Build history of the part. All positions in model axes, mm. Give positions to 0.01 mm unless a question says otherwise; leave off trailing zeros. Write each loop counter-clockwise with the first axis right and the second up, starting at its lowest first coordinate (ties: lowest second). Pieces come first, ordered by that corner, then holes. Notation, with made-up numbers: M 85,-21.5 L 138,-21.5 A21 ccw 138,-0.5 Z; hole C 6.5,9 d5. An arc over 180 degrees is marked long. Return JSON: item names as keys, results as strings. Group by question number.
Q1. Band-saw the part on A-A, the plane y = 0. Give the cut face in (x, z), then the cut area to 4 significant figures.
Q2. Band-saw the part on D-D, the plane y = -30. Give the cut face in (x, z), then the cut area to 3 significant figures.
Q3. Wall check: probe 1 along Y at (x, z) = (163.5, 0); probe 2 along Z at (x, y) = (209.5, -2). Give the ranges that are in metal, low to high.
Q4. Flat gauge pins, fed straight in: pin 1 Ø6 at (y, z) = (-29, -20.5) entering from -X; pin 2 Ø10 at (x, z) = (-243.5, 9) entering from +Y; pin 3 Ø2 at (x, z) = (120, -12) entering from +Y. Where does each tip first touch, or does it go through?
Q5. Pull direction Z, two halves, no side cores. Call faces 1 (the flat face through (-305, 17, 8)), 2 (the flat face through (-275, 1, -1)), 3 (the cylindrical face through (-317.325, 13.887, -10.648)), 4 (the cylindrical face through (19.06, -8.02, 36.12)): +Z half, -Z half, draft (parallel to the pull), parting line (faces both ways), or undercut.
Q6. Band-saw the part on C-C, the plane x = -163.5. Give the cut face in (y, z).
from build123d import *

# Parameters (mm, degrees)
F0_W     = 30
F0_H     = 37
F2_R     = 17.5
F3_DEPTH = 25


with BuildPart() as f1:
    # F0 (on Top) → F1 (revolve)
    with BuildSketch(Plane.XY):
        Polygon((305, 40), (-305, 40), (-305, 37), (-275, 37), (305, 37), align=None)
        with Locations((-290, 18.5)):
            Rectangle(F0_W, F0_H)
    revolve(axis=Axis((-46.437122, 0, 0), (-1, 0, 0)))

    # F2 (on face) → F3 (join)
    with BuildSketch(Plane(origin=(-305, 0, 0), x_dir=(0, -1, 0), z_dir=(-1, 0, 0))):
        Circle(F2_R)
    extrude(amount=F3_DEPTH)


solid = f1.part
From the geometry:
{
 "1": {"outline": "M -330,-17.5 L -305,-17.5 L -305,-40 L 305,-40 L 305,-37 L -275,-37 L -275,37 L 305,37 L 305,40 L -305,40 L -305,17.5 L -330,17.5 Z", "area": "6,755 mm^2"},
 "2": {"outline": "M -305,-26.46 L 305,-26.46 L 305,-21.66 L -275,-21.66 L -275,21.66 L 305,21.66 L 305,26.46 L -305,26.46 Z", "area": "7,160 mm^2"},
 "3": {"probe 1": "y = -40 to -37, 37 to 40", "probe 2": "z = -39.95 to -36.95, 36.95 to 39.95"},
 "4": {"pin 1": "stops at x = -305", "pin 2": "stops at y = 39.8", "pin 3": "stops at y = 38.46"},
 "5": {"face 1": "draft", "face 2": "undercut", "face 3": "parting line", "face 4": "undercut"},
 "6": {"outline": "C 0,0 d80; hole C 0,0 d74"}
}
